The model under review builds one solid part; all positions refer to its coordinate system, in mm. A direction names the side the tool comes from. Round coordinates to 2 decimals unless told otherwise and drop trailing zeros. Order: outer loops, then holes, each group sorted by start corner. A loop starts at its lowest first (then second) coordinate and runs counter-clockwise, first axis right, second up. Notation, with made-up numbers: (69, -18) -> (125, -18) arc R12 cw to (125, 0) -> close; hole circle Ø4 at (45, 88). An arc over 180 degrees is marked (long way). Return JSON: item names as keys, results as strings. Group by question number.
from build123d import *

# Parameters (mm, degrees)
SKETCH1_W           = 14
SKETCH1_H           = 54
BOSS_EXTRUDE2_DEPTH = 35
SHELL2_T            = -5
SKETCH2_W           = 54
SKETCH2_H           = 2
BOSS_EXTRUDE3_DEPTH = 12
SKETCH3_W           = 54
SKETCH3_H           = 2
BOSS_EXTRUDE4_DEPTH = 12


with BuildPart() as part:
    # Sketch1 → Boss-Extrude2 (new body)
    with BuildSketch(Plane(origin=(0, 0, 0), x_dir=(1, 0, 0), z_dir=(0, 1, 0))):
        with Locations((7, 27)):
            Rectangle(SKETCH1_W, SKETCH1_H)
    extrude(amount=BOSS_EXTRUDE2_DEPTH)

    # Shell2
    shell2_openings = [part.faces().sort_by_distance(p)[0] for p in [
        (7, 0, -27),
    ]]
    offset(amount=SHELL2_T, openings=shell2_openings, kind=Kind.INTERSECTION)

    # Sketch2 → Boss-Extrude3 (add)
    with BuildSketch(Plane.ZY):
        with Locations((-27, 34)):
            Rectangle(SKETCH2_W, SKETCH2_H)
    extrude(amount=BOSS_EXTRUDE3_DEPTH)

    # Sketch3 → Boss-Extrude4 (add)
    with BuildSketch(Plane(origin=(14, 0, 0), x_dir=(0, 0, -1), z_dir=(1, 0, 0))):
        with Locations((27, 34)):
            Rectangle(SKETCH3_W, SKETCH3_H)
    extrude(amount=BOSS_EXTRUDE4_DEPTH)


solid = part.part
Item 1: Consider section A-A on z = -50.5. State the section outline as (x, y) points, plus the area to 3 significant figures.
Item 2: Consider section C-C on z = -29. State the section outline as (x, y) points.
Item 3: Consider section B-B on y = 16. State the section outline as (x, z) points, plus the area to 3 significant figures.
Item 4: For faces 4 (the face through (0, 16, -27)), 5 (the face through (14, 16, -27)), 6 (the face through (7, 15, -49)), list the 3-axis set-ups (+Z, -Z, +X, -X, +Y, -Y) from which the entire face can be reached by the end or side of a thin tool; tool diameter is ignored.
Item 5: Insertion check: pin 1 Ø4.5 at (x, y) = (7, 19.5) entering from +Z; pin 2 Ø6 at (x, z) = (-9, -27.5) entering from -Y; pin 3 Ø10 at (y, z) = (24, -36.5) entering from -X; pin 4 Ø1.2 at (x, z) = (7.5, -32.5) entering from -Y. Each pin has a flat end and moves straight along its axis. Give the tip position at first contact, or say it passes through.
Item 6: The part is to be moulded in two halves that separate along X. For faces 1 (the face through (7, 30, -27)), 2 (the face through (-12, 34, -27)), 3 (the face through (-6, 33, -27)), say which applies: +X half, -X half, draft (parallel to the pull), parting line (faces both ways), or undercut.
Item 7: Wall thickness on line 1 along X through (y, z) = (9, -45.5); line 2 along Z through (x, y) = (7, 15.5); line 3 along Y through (x, z) = (21.5, -52): over which ranges is each line inside the solid? List them lowest first.
Item 8: Consider section D-D on x = -3. State the section outline as (y, z) points, plus the area to 3 significant figures.
Values:
{
 "1": {"outline": "(-12, 33) -> (0, 33) -> (0, 0) -> (14, 0) -> (14, 33) -> (26, 33) -> (26, 35) -> (-12, 35) -> close", "area": "538 mm^2"},
 "2": {"outline": "(-12, 33) -> (0, 33) -> (0, 0) -> (5, 0) -> (5, 30) -> (9, 30) -> (9, 0) -> (14, 0) -> (14, 33) -> (26, 33) -> (26, 35) -> (-12, 35) -> close"},
 "3": {"outline": "(0, -54) -> (14, -54) -> (14, 0) -> (0, 0) -> close; hole (5, -49) -> (9, -49) -> (9, -5) -> (5, -5) -> close", "area": "580 mm^2"},
 "4": {"face 4": "+Z, -Z, -X, -Y", "face 5": "+Z, -Z, +X, -Y", "face 6": "-Y"},
 "5": {"pin 1": "z = 0", "pin 2": "y = 33", "pin 3": "x = 0", "pin 4": "y = 30"},
 "6": {"face 1": "undercut", "face 2": "-X half", "face 3": "draft"},
 "7": {"line 1": "0 to 5, 9 to 14", "line 2": "-54 to -49, -5 to 0", "line 3": "33 to 35"},
 "8": {"outline": "(33, -54) -> (35, -54) -> (35, 0) -> (33, 0) -> close", "area": "108 mm^2"}
}
